Autodesk Inventor part; units mm, degrees
ref_plane "YZ Plane" through (0, 0, 0) normal (1, 0, 0) x (0, 1, 0)
ref_plane "XZ Plane" through (0, 0, 0) normal (0, 1, 0) x (-1, 0, 0)
ref_plane "XY Plane" through (0, 0, 0) normal (0, 0, 1) x (1, 0, 0)
sketch "Sketch1" plane through (0, 0, 0) normal (0, 1, 0) x (-1, 0, 0)
  line L0 (0, 0) -> (0, 38.5027)
  line L1 (0, 38.5027) -> (-13.5, 27.1748)
  line L2 (-13.5, 27.1748) -> (-13.5, 50.6722)
  line L3 (-13.5, 50.6722) -> (0, 62)
  line L4 (0, 62) -> (18, 62)
  line L5 (18, 62) -> (18, 0)
  line L6 (18, 0) -> (31.5, 0)
  line L7 (31.5, 0) -> (31.5, -18)
  line L8 (31.5, -18) -> (-13.5, -18)
  line L9 (-13.5, -18) -> (-13.5, 0)
  line L10 (-13.5, 0) -> (0, 0)
  dimension "d0" = 50
  dimension "d1" = 80
  dimension "d2" = 18
  dimension "d3" = 18
  dimension "d4" = 13.5
  dimension "d5" = 13.5
  dimension "d6" = 18
  dimension "d7" = 0
  dimension "d8" = 0
  dimension "d9" = 0
extrude "Extrusion1" add sketch "Sketch1" along normal blind 18
fillet "Fillet1" radius 2 3 edges at (-18, 9, 62) (0, 9, 62) (13.5, 9, 50.6722)
fillet "Fillet2" radius 1 2 edges at (0, 9, 38.5027) (13.5, 9, 27.1748)
fillet "Fillet3" radius 4 6 edges at (13.5, 9, 0) (13.5, 9, -18) (-31.5, 9, -18) (-18, 9, 0) (-31.5, 9, 0) (0, 9, 0)
sketch "Sketch2" plane through (0, 18, 0) normal (0, 1, 0) x (1, 0, 0)
  line L0 (-16, -62) -> (-0.7279, -62)
  line L1 (-4, 2) -> (-14, 2)
  line L2 (-14, -6) -> (-14, 2)
  line L3 (-4, 2) -> (-4, -6)
  line L4 (-4, -6) -> (-6, -6)
  line L5 (-6, -6) -> (-6, 0)
  line L6 (-6, 0) -> (-12, 0)
  line L7 (-12, 0) -> (-12, -6)
  line L8 (-12, -6) -> (-14, -6)
  line L9 (-4, -8) -> (-14, -8)
  line L10 (-14, -8) -> (-14, -16)
  line L11 (-12, -16) -> (-14, -16)
  line L12 (-12, -16) -> (-12, -10)
  line L13 (-12, -10) -> (-10, -10)
  line L14 (-10, -10) -> (-10, -14)
  line L15 (-10, -14) -> (-8, -14)
  line L16 (-8, -14) -> (-8, -10)
  line L17 (-8, -10) -> (-6, -10)
  line L18 (-6, -10) -> (-6, -16)
  line L19 (-6, -16) -> (-4, -16)
  line L20 (-4, -8) -> (-4, -16)
  line L21 (-4, -18) -> (-10, -18)
  line L22 (-10, -18) -> (-10, -24)
  line L23 (-10, -24) -> (-12, -24)
  line L24 (-12, -24) -> (-12, -18)
  line L25 (-12, -18) -> (-14, -18)
  line L26 (-14, -18) -> (-14, -26)
  line L27 (-14, -26) -> (-8, -26)
  line L28 (-8, -26) -> (-8, -20)
  line L29 (-8, -20) -> (-6, -20)
  line L30 (-6, -20) -> (-6, -26)
  line L31 (-6, -26) -> (-4, -26)
  line L32 (-4, -18) -> (-4, -26)
  line L33 (-4, -28) -> (-14, -28)
  line L34 (-14, -36) -> (-4, -36)
  line L35 (-4, -36) -> (-4, -28)
  line L36 (-6, -30) -> (-10, -30)
  line L37 (-10, -30) -> (-10, -34)
  line L38 (-4, -38) -> (-14, -38)
  line L39 (-1, -19.7264) -> (-2.5, -12)
  line L40 (-4, -6) -> (-4, -8) construction
  line L41 (-4, -16) -> (-4, -18) construction
  line L42 (-4, -26) -> (-4, -28) construction
  line L43 (-4, -36) -> (-4, -38) construction
  line L44 (-14, -36) -> (-14, -38) construction
  line L45 (-14, -6) -> (-14, -8) construction
  line L46 (-14, -26) -> (-14, -28) construction
  line L47 (-6, -26) -> (-8, -26) construction
  line L48 (-10, -18) -> (-12, -18) construction
  line L49 (-8, -20) -> (-8, -18) construction
  line L50 (-10, -24) -> (-8, -24) construction
  line L51 (-10, -24) -> (-10, -26) construction
  line L52 (-6, -10) -> (-6, -8) construction
  line L53 (-12, -30) -> (-14, -30)
  line L54 (-14, -30) -> (-14, -28)
  line L55 (-14, -34) -> (-14, -36)
  line L56 (-6, -30) -> (-6, -28) construction
  line L57 (-6, -30) -> (-6, -34)
  line L58 (-6, -34) -> (-6, -36) construction
  line L59 (-6, -30) -> (-4, -30) construction
  line L60 (-12, -30) -> (-12, -34)
  line L61 (-12, -34) -> (-14, -34)
  line L62 (-10, -30) -> (-12, -30) construction
  line L63 (-4, -38) -> (-4, -46)
  line L64 (-6, -40) -> (-6, -38) construction
  line L65 (-6, -40) -> (-4, -40) construction
  line L66 (-14, -38) -> (-14, -41)
  line L67 (-14, -41) -> (-12, -41)
  line L68 (-12, -41) -> (-14, -43)
  line L69 (-14, -43) -> (-14, -46)
  line L70 (-14, -46) -> (-12, -44)
  line L71 (-12, -44) -> (-12, -46)
  line L72 (-12, -46) -> (-4, -46)
  line L73 (-10, -40) -> (-10, -44)
  line L74 (-10, -44) -> (-6, -44)
  line L75 (-6, -44) -> (-6, -40)
  line L76 (-2.5, -12) -> (-1, -13.7264)
  line L77 (-12, -46) -> (-14, -46) construction
  line L78 (-14, -41) -> (-14, -43) construction
  line L79 (-6, -40) -> (-10, -40)
  line L80 (-10, -44) -> (-12, -44) construction
  line L81 (-14, -16) -> (-14, -18) construction
  line L82 (-6, -34) -> (-10, -34)
  line L83 (-1, -13.7264) -> (-1, -19.7264)
  line L84 (-1, -13.7264) -> (-1, -12) construction
  line L85 (-1, -12) -> (-2.5, -12) construction
  line L86 (-2.5, -12) -> (-4, -12) construction
  line L87 (-18, -4) -> (-18, -60)
  line L88 (0, -36.3582) -> (0, -4)
  line L89 (9.5, 18) -> (-27.5, 18)
  line L90 (-9, -46) -> (-9, -62) construction
  line L91 (-9, 2) -> (-9, 18) construction
  line L92 (-4, -22) -> (0, -22) construction
  line L93 (-14, -22) -> (-18, -22) construction
  point P0 (0, 0)
  dimension "d18" = 10
  dimension "d19" = 8
  dimension "d20" = 2
  dimension "d21" = 45
  dimension "d26" = 0
  dimension "d29" = 3
  dimension "d31" = 30
extrude "Extrusion2" cut sketch "Sketch2" against normal blind 3
Geometry: final body of the model. Coordinates: model frame, mm. A direction names the side the tool comes from. Round coordinates to 2 decimals unless told otherwise and drop trailing zeros. Loops run counter-clockwise (first coordinate to the right, second up) from the corner with the lowest first, then second, coordinate; pieces in that order, holes last.
Q1. Section B-B on y = 12. Return loops of the section in (x, z).
Q2. Access query for faces 5 (the flat face through (6.76, 8.87, 56.33)), 6 (the flat face through (-11, 17, 10)). Directions: +Z, -Z, +X, -X, +Y, -Y. A direction counts if a zero-diameter tool reaches every point of the face in a straight line with its end or side. Return the directions, or none.
Q3. Material intervals for L1, parallel to X at y = 17.25, z = 5; L2, parallel to X at y = 1.75, z = 5; L3, parallel to X at y = 16.75, z = 44.5, sorted ascending.
Q4. Pull-direction query (Z, two-part tool) for faces 1 (the cylindrical face through (-19.141, 9.126, 1.203)), 2 (the flat face through (-13, 17, 30)), 3 (the cylindrical face through (12.359, 9.126, -16.797)), 4 (the flat face through (-14, 17, 44)); classes: released by +Z, released by -Z, zero draft, split by the parting line, or undercut.
Q5. Section C-C on x = 5. Return loops of the section in (y, z), plus the area to 3 significant figures.
Q6. Section A-A on z = 32. Return loops of the section in (x, y).
Q7. Section D-D on x = -26. Return loops of the section in (y, z), plus the area to 3 significant figures.
Q8. Pin query (flat end, axial travel): P1, Ø0.9, axis at y = 16, z = 12, coming from the +X side; P2, Ø3.5, axis at y = 16.5, z = 4, coming from the -X side; P3, Ø1.5, axis at y = 16, z = 21.5, coming from the -X side. Return the tip coordinate at first contact, or that it passes through.
Evaluation:
1. outline: (-31.5, -14) arc R4 ccw to (-27.5, -18) - (9.5, -18) arc R4 ccw to (13.5, -14) - (13.5, -4) arc R4 ccw to (9.5, 0) - (4, 0) arc R4 cw to (0, 4) - (0, 36.36) arc R1 cw to (1.64, 37.12) - (11.86, 28.55) arc R1 ccw to (13.5, 29.32) - (13.5, 49.74) arc R2 ccw to (12.79, 51.27) - (0.56, 61.53) arc R2 ccw to (-0.73, 62) - (-16, 62) arc R2 ccw to (-18, 60) - (-18, 4) arc R4 cw to (-22, 0) - (-27.5, 0) arc R4 ccw to (-31.5, -4) - close
2. face 5: +Z, +X, +Y, -Y
2. face 6: +Y
3. L1: x = -18 to -14, -12 to -6, -4 to 0
3. L2: x = -18 to 0
3. L3: x = -18 to -14, -12.5 to -12, -4 to 13.5
4. face 1: released by +Z
4. face 2: undercut
4. face 3: released by -Z
4. face 4: undercut
5. outline: (0, -18) - (18, -18) - (18, 0) - (0, 0) - close; (0, 34.31) - (18, 34.31) - (18, 57.8) - (0, 57.8) - close
5. area: 747 mm2
6. outline: (-18, 0) - (0, 0) - (0, 18) - (-4, 18) - (-4, 15) - (-6, 15) - (-6, 18) - (-10, 18) - (-10, 15) - (-12, 15) - (-12, 18) - (-18, 18) - close; (7.75, 0) - (13.5, 0) - (13.5, 18) - (7.75, 18) - close
7. outline: (0, -18) - (18, -18) - (18, 0) - (0, 0) - close
7. area: 324 mm2
8. P1: stops at x = 0
8. P2: stops at x = -18.4
8. P3: stops at x = -18
